```python
from build123d import *

# Parameters (mm, degrees)
SKETCH1_R           = 49.0728
SKETCH1_R_2         = 45.5676
EXTRUDE_THIN1_DEPTH = 17.3482
SKETCH2_R           = 22.9489
SKETCH2_R_2         = 18.9103
BOSS_EXTRUDE1_DEPTH = 2.8702
SKETCH3_R           = 48.26
SKETCH3_R_2         = 12.8778
BOSS_EXTRUDE2_DEPTH = 2.5654
CHAMFER1_SIZE       = 2.54
SKETCH4_W           = 10.0838
SKETCH4_H           = 6.023980684
CUT_EXTRUDE1_DEPTH  = 1.0668
CUT_EXTRUDE2_START  = -1.651
CUT_EXTRUDE2_DEPTH  = 1.651
CUT_EXTRUDE3_DEPTH  = 5.3594


with BuildPart() as part:
    # Sketch1 → Extrude-Thin1 (new body)
    with BuildSketch(Plane(origin=(0, 0, 0), x_dir=(1, 0, 0), z_dir=(0, 1, 0))):
        Circle(SKETCH1_R)
        Circle(SKETCH1_R_2, mode=Mode.SUBTRACT)
    extrude(amount=EXTRUDE_THIN1_DEPTH)



with BuildPart() as body_2:
    # Sketch2 → Boss-Extrude1 (new body)
    # profile 1 of 11: a face of its own
    with BuildSketch(Plane.XZ):
        Circle(SKETCH2_R)
        with Locations(Location((0, 0, 0), (0, 0, 270))):
            Circle(SKETCH2_R_2, mode=Mode.SUBTRACT)
    # profile 2 of 11: a face of its own
    with BuildSketch(Plane.XZ):
        with BuildLine():
            ThreePointArc((-21.14191931, -8.925875818), (-21.825700887, -7.091600102), (-22.350670185, -5.205723149))
            Line((-22.350670185, -5.205723149), (-43.901801922, -12.208110326))
            ThreePointArc((-43.901801922, -12.208110326), (-43.337362912, -14.081162793), (-42.693051047, -15.928262996))
            Line((-42.693051047, -15.928262996), (-21.14191931, -8.925875818))
        make_face()
    # profile 3 of 11: a face of its own
    with BuildSketch(Plane.XZ):
        with BuildLine():
            ThreePointArc((-22.350670185, 5.205723149), (-21.825700887, 7.091600102), (-21.14191931, 8.925875818))
            Line((-21.14191931, 8.925875818), (-42.693051047, 15.928262996))
            ThreePointArc((-42.693051047, 15.928262996), (-43.337362912, 14.081162793), (-43.901801922, 12.208110326))
            Line((-43.901801922, 12.208110326), (-22.350670185, 5.205723149))
        make_face()
    # profile 4 of 11: a face of its own
    with BuildSketch(Plane.XZ):
        with BuildLine():
            ThreePointArc((-11.857673846, -19.648093602), (-13.489024976, -18.566050102), (-15.022224721, -17.348912809))
            Line((-15.022224721, -17.348912809), (-28.34155663, -35.681400442))
            ThreePointArc((-28.34155663, -35.681400442), (-26.783963262, -36.864962793), (-25.177005755, -37.980581235))
            Line((-25.177005755, -37.980581235), (-11.857673846, -19.648093602))
        make_face()
    # profile 5 of 11: a face of its own
    with BuildSketch(Plane.XZ):
        with BuildLine():
            ThreePointArc((1.9558, -22.865407444), (0, -22.9489), (-1.9558, -22.865407444))
            Line((-1.9558, -22.865407444), (-1.9558, -45.525608355))
            ThreePointArc((-1.9558, -45.525608355), (0, -45.5676), (1.9558, -45.525608355))
            Line((1.9558, -45.525608355), (1.9558, -22.865407444))
        make_face()
    # profile 6 of 11: a face of its own
    with BuildSketch(Plane.XZ):
        with BuildLine():
            Line((28.34155663, -35.681400442), (15.022224721, -17.348912809))
            ThreePointArc((15.022224721, -17.348912809), (13.489024976, -18.566050102), (11.857673846, -19.648093602))
            Line((11.857673846, -19.648093602), (25.177005755, -37.980581235))
            ThreePointArc((25.177005755, -37.980581235), (26.783963262, -36.864962793), (28.34155663, -35.681400442))
        make_face()
    # profile 7 of 11: a face of its own
    with BuildSketch(Plane.XZ):
        with BuildLine():
            Line((43.901801922, -12.208110326), (22.350670185, -5.205723149))
            ThreePointArc((22.350670185, -5.205723149), (21.825700887, -7.091600102), (21.14191931, -8.925875818))
            Line((21.14191931, -8.925875818), (42.693051047, -15.928262996))
            ThreePointArc((42.693051047, -15.928262996), (43.337362912, -14.081162793), (43.901801922, -12.208110326))
        make_face()
    # profile 8 of 11: a face of its own
    with BuildSketch(Plane.XZ):
        with BuildLine():
            Line((42.693051047, 15.928262996), (21.14191931, 8.925875818))
            ThreePointArc((21.14191931, 8.925875818), (21.825700887, 7.091600102), (22.350670185, 5.205723149))
            Line((22.350670185, 5.205723149), (43.901801922, 12.208110326))
            ThreePointArc((43.901801922, 12.208110326), (43.337362912, 14.081162793), (42.693051047, 15.928262996))
        make_face()
    # profile 9 of 11: a face of its own
    with BuildSketch(Plane.XZ):
        with BuildLine():
            Line((25.177005755, 37.980581235), (11.857673846, 19.648093602))
            ThreePointArc((11.857673846, 19.648093602), (13.489024976, 18.566050102), (15.022224721, 17.348912809))
            Line((15.022224721, 17.348912809), (28.34155663, 35.681400442))
            ThreePointArc((28.34155663, 35.681400442), (26.783963262, 36.864962793), (25.177005755, 37.980581235))
        make_face()
    # profile 10 of 11: a face of its own
    with BuildSketch(Plane.XZ):
        with BuildLine():
            ThreePointArc((-15.022224721, 17.348912809), (-13.489024976, 18.566050102), (-11.857673846, 19.648093602))
            Line((-11.857673846, 19.648093602), (-25.177005755, 37.980581235))
            ThreePointArc((-25.177005755, 37.980581235), (-26.783963262, 36.864962793), (-28.34155663, 35.681400442))
            Line((-28.34155663, 35.681400442), (-15.022224721, 17.348912809))
        make_face()
    # profile 11 of 11: a face of its own
    with BuildSketch(Plane.XZ):
        with BuildLine():
            Line((-1.9558, 45.525608355), (-1.9558, 22.9489))
            Line((-1.9558, 22.9489), (-1.9558, 22.865407444))
            ThreePointArc((-1.9558, 22.865407444), (0, 22.9489), (1.9558, 22.865407444))
            Line((1.9558, 22.865407444), (1.9558, 22.9489))
            Line((1.9558, 22.9489), (1.9558, 45.525608355))
            ThreePointArc((1.9558, 45.525608355), (0, 45.5676), (-1.9558, 45.525608355))
        make_face()
    extrude(amount=-BOSS_EXTRUDE1_DEPTH)


with BuildPart() as part_1:
    add(part.part)

    add(body_2.part)  # Boss-Extrude2 merges body 2
    # Sketch3 → Boss-Extrude2 (add)
    with BuildSketch(Plane(origin=(0, 2.8702, 0), x_dir=(1, 0, 0), z_dir=(0, 1, 0))):
        Circle(SKETCH3_R)
        with Locations(Location((0, 0, 0), (0, 0, 270))):
            Circle(SKETCH3_R_2, mode=Mode.SUBTRACT)
    extrude(amount=BOSS_EXTRUDE2_DEPTH)

    # Chamfer1
    chamfer1_edges = [part_1.edges().sort_by_distance(p)[0] for p in [
        (0, 5.4356, -12.8778),
    ]]
    chamfer(chamfer1_edges, length=CHAMFER1_SIZE)

    # Sketch4 → Cut-Extrude1 (cut)
    with BuildSketch(Plane.XZ.offset(-2.8702)):
        with Locations((0, 14.323509658)):
            Rectangle(SKETCH4_W, SKETCH4_H)
    extrude(amount=-CUT_EXTRUDE1_DEPTH, mode=Mode.SUBTRACT)

    # Sketch6 → Cut-Extrude2 (cut)
    with BuildSketch(Plane(origin=(0, 5.4356, 0), x_dir=(1, 0, 0), z_dir=(0, 1, 0)).offset(CUT_EXTRUDE2_START)):
        with BuildLine():
            ThreePointArc((-16.056697944, -10.381176076), (-17.664865749, -7.317026971), (-18.6944, -4.0132))
            Line((-18.6944, -4.0132), (-45.38377728, -4.088878764))
            ThreePointArc((-45.38377728, -4.088878764), (-42.098972986, -17.437965573), (-34.982450572, -29.19990277))
            Line((-34.982450572, -29.19990277), (-16.056697944, -10.381176076))
        make_face()
        with BuildLine():
            ThreePointArc((-4.0132, -18.6944), (-7.317026971, -17.664865749), (-10.381176076, -16.056697944))
            Line((-10.381176076, -16.056697944), (-29.19990277, -34.982450572))
            ThreePointArc((-29.19990277, -34.982450572), (-17.437965573, -42.098972986), (-4.088878764, -45.38377728))
            Line((-4.088878764, -45.38377728), (-4.0132, -18.6944))
        make_face()
        with BuildLine():
            Line((29.19990277, -34.982450572), (10.381176076, -16.056697944))
            ThreePointArc((10.381176076, -16.056697944), (7.317026971, -17.664865749), (4.0132, -18.6944))
            Line((4.0132, -18.6944), (4.088878764, -45.38377728))
            ThreePointArc((4.088878764, -45.38377728), (17.437965573, -42.098972986), (29.19990277, -34.982450572))
        make_face()
        with BuildLine():
            Line((45.383730316, -4.0894), (18.677879249, -4.0894))
            ThreePointArc((18.677879249, -4.0894), (17.649910049, -7.353029366), (16.056697944, -10.381176076))
            Line((16.056697944, -10.381176076), (34.982450572, -29.19990277))
            ThreePointArc((34.982450572, -29.19990277), (42.098872847, -17.438207328), (45.383730316, -4.0894))
        make_face()
        with BuildLine():
            Line((34.982450572, 29.19990277), (16.056697944, 10.381176076))
            ThreePointArc((16.056697944, 10.381176076), (17.664865749, 7.317026971), (18.6944, 4.0132))
            Line((18.6944, 4.0132), (45.38377728, 4.088878764))
            ThreePointArc((45.38377728, 4.088878764), (42.098972986, 17.437965573), (34.982450572, 29.19990277))
        make_face()
        with BuildLine():
            ThreePointArc((29.19990277, 34.982450572), (17.437965573, 42.098972986), (4.088878764, 45.38377728))
            Line((4.088878764, 45.38377728), (4.0132, 18.6944))
            ThreePointArc((4.0132, 18.6944), (7.317026971, 17.664865749), (10.381176076, 16.056697944))
            Line((10.381176076, 16.056697944), (29.19990277, 34.982450572))
        make_face()
        with BuildLine():
            Line((-4.0132, 18.6944), (-4.088878764, 45.38377728))
            ThreePointArc((-4.088878764, 45.38377728), (-17.437965573, 42.098972986), (-29.19990277, 34.982450572))
            Line((-29.19990277, 34.982450572), (-10.381176076, 16.056697944))
            ThreePointArc((-10.381176076, 16.056697944), (-7.317026971, 17.664865749), (-4.0132, 18.6944))
        make_face()
        with BuildLine():
            ThreePointArc((-18.6944, 4.0132), (-17.664865749, 7.317026971), (-16.056697944, 10.381176076))
            Line((-16.056697944, 10.381176076), (-34.982450572, 29.19990277))
            ThreePointArc((-34.982450572, 29.19990277), (-42.098972986, 17.437965573), (-45.38377728, 4.088878764))
            Line((-45.38377728, 4.088878764), (-18.6944, 4.0132))
        make_face()
    extrude(amount=CUT_EXTRUDE2_DEPTH, mode=Mode.SUBTRACT)

    # Sketch7 → Cut-Extrude3 (cut)
    with BuildSketch(Plane(origin=(0, 17.3482, 0), x_dir=(1, 0, 0), z_dir=(0, 1, 0))):
        with BuildLine():
            Line((-45.399557639, 3.175), (-45.399557639, -3.175))
            ThreePointArc((-45.399557639, -3.175), (-46.72329814, 0), (-45.399557639, 3.175))
        make_face()
        with BuildLine():
            Line((45.3995595, -3.175), (45.3995595, 3.175))
            ThreePointArc((45.3995595, 3.175), (46.7233, 0), (45.3995595, -3.175))
        make_face()
    extrude(amount=-CUT_EXTRUDE3_DEPTH, mode=Mode.SUBTRACT)


solid = part_1.part
```
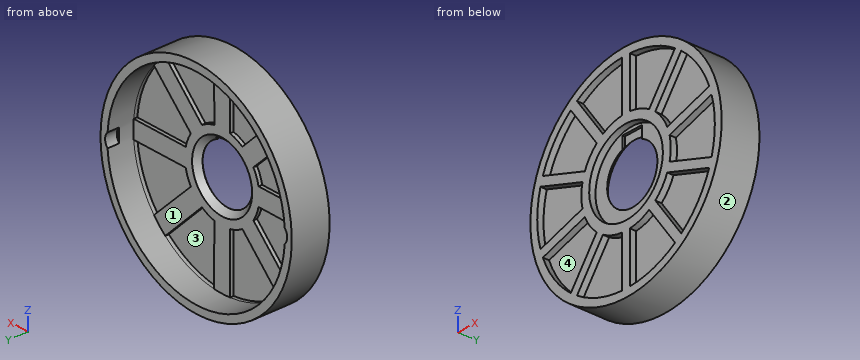
CAD build for the part. Positions are in the model's coordinates, mm. Face numbers are marked on the shaded views. A direction names the side the tool comes from. Coordinates: 2 decimals unless noted, no trailing zeros. Loops run counter-clockwise (first coordinate to the right, second up) from the corner with the lowest first, then second, coordinate; pieces in that order, holes last. Notation, with made-up numbers: (29, 24) - (33, 24) arc R12 ccw to (33, 37) - close; hole circle Ø9 at (-29, 51.25). An arc over 180 degrees is marked (long way). Return JSON: item names as keys, results as strings.
1. Drop flat-ended pins along their axis: pin 1 (8 mm diameter, centred on y = 9.5, z = -4.5, fed in from +X); pin 2 (6 mm diameter, centred on x = -15.5, y = 6.5, fed in from -Z); pin 3 (8 mm diameter, centred on x = 1, y = 13, fed in from +Z). Give the stop position or say it passes through.
Result:
{"pin 1": "stops at x = 49.07", "pin 2": "stops at z = -47.45", "pin 3": "stops at z = 49.07"}
2. Band-saw the part on D-D (z = 40.5). Give the cut face in (x, y), and give its area (3 significant figures).
Result:
{"outline": "(-27.71, 0) - (-20.88, 0) - (-20.88, 2.87) - (-1.96, 2.87) - (-1.96, 0) - (1.96, 0) - (1.96, 2.87) - (20.88, 2.87) - (20.88, 0) - (27.71, 0) - (27.71, 17.35) - (20.88, 17.35) - (20.88, 3.78) - (4.08, 3.78) - (4.08, 5.44) - (-4.08, 5.44) - (-4.08, 3.78) - (-20.88, 3.78) - (-20.88, 17.35) - (-27.71, 17.35) - close", "area": "300 mm2"}
3. Mould opens along X. For the marked faces 1 and 2 say: released by +X, released by -X, zero draft, split by the parting line, or undercut.
Result:
{"face 1": "undercut", "face 2": "split by the parting line"}
4. 3-axis set-ups, long thin cutter, end or side, ignore diameter. For the marked faces 3 and 4: which of +Z, -Z, +X, -X, +Y, -Y reach the whole face in a straight line?
Result:
{"face 3": "+Y", "face 4": "-Y"}
5. Probe L1, parallel to X at y = 1.2, z = 0; L2, parallel to X at y = 11, z = 0; L3, parallel to Z at x = 6, y = 2.25. List the from-to ranges inside material, lowest first. Write a range as from..to.
Result:
{"L1": "x = -49.07..-45.57, -22.95..-18.91, 18.91..22.95, 45.57..49.07", "L2": "x = -49.07..-45.57, 45.57..49.07", "L3": "z = -48.7..-45.17, -22.15..-17.93, 17.93..22.15, 45.17..48.7"}
